Autodesk Inventor part; units mm, degrees
ref_plane "YZ Plane" through (0, 0, 0) normal (1, 0, 0) x (0, 1, 0)
ref_plane "XZ Plane" through (0, 0, 0) normal (0, 1, 0) x (-1, 0, 0)
ref_plane "XY Plane" through (0, 0, 0) normal (0, 0, 1) x (1, 0, 0)
sketch "Эскиз1" plane through (0, 0, 0) normal (0, 1, 0) x (-1, 0, 0)
  line L0 (0, 0) -> (-19.5, 0)
  line L1 (-19.5, 0) -> (-19.5, -40.5)
  line L2 (-19.5, -40.5) -> (0, -40.5)
  line L3 (0, -40.5) -> (0, 0)
  line L4 (-19.5, -40.5) -> (-19.5, -45.5)
  line L5 (-19.5, -45.5) -> (-15, -45.5)
  line L6 (0, -45.5) -> (-4.5, -45.5)
  line L7 (-4.5, -45.5) -> (-15, -45.5)
  line L8 (0, -40.5) -> (-19.5, -40.5)
  line L9 (-19.5, -40.5) -> (-19.5, -50.5)
  line L10 (-19.5, -50.5) -> (0, -50.5)
  line L11 (0, -50.5) -> (0, -40.5)
  line L12 (0, 0) -> (-19.5, 0)
  line L13 (-19.5, 0) -> (-19.5, 10)
  line L14 (-19.5, 10) -> (0, 10)
  line L15 (0, 10) -> (0, 0)
  line L16 (0, 5) -> (-4.5, 5)
  line L17 (-4.5, 5) -> (-15, 5)
  line L18 (-15, 5) -> (-19.5, 5)
  line L19 (-19.5, -50.5) -> (-23.5, -50.5)
  line L20 (-23.5, -50.5) -> (-23.5, 10)
  line L21 (-23.5, 10) -> (-19.5, 10)
  line L22 (-19.5, 10) -> (-19.5, -50.5)
  line L23 (0, 10) -> (4, 10)
  line L24 (4, 10) -> (4, -50.5)
  line L25 (4, -50.5) -> (0, -50.5)
  line L26 (0, -50.5) -> (0, 10)
  circle A0 centre (-4.5, -45.5) radius 1.25
  circle A1 centre (-15, -45.5) radius 1.25
  circle A2 centre (-4.5, 5) radius 1.25
  circle A3 centre (-15, 5) radius 1.25
  circle A4 centre (0, -40.5) radius 0.5
  circle A5 centre (-19.5, -40.5) radius 0.5
  circle A6 centre (0, 0) radius 0.5
  circle A7 centre (-19.5, 0) radius 0.5
  point P0 (-19, 0)
  point P1 (-0.5, 0)
  point P2 (0, -0.5)
  point P3 (0, -40)
  point P4 (-0.5, -40.5)
  point P5 (-19, -40.5)
  point P6 (-19.5, -40)
  point P7 (-19.5, -0.5)
  dimension "d0" = 19.5
  dimension "d1" = 40.5
  dimension "d2" = 5
  dimension "d3" = 4.5
  dimension "d4" = 4.5
  dimension "d5" = 10
  dimension "d6" = 10
  dimension "d7" = 4
  dimension "d8" = 4
  dimension "d9" = 2.5
  dimension "d10" = 2.5
  dimension "d11" = 2.5
  dimension "d12" = 2.5
  dimension "d16" = 1
  dimension "d17" = 1
  dimension "d18" = 1
  dimension "d19" = 1
extrude "Выдавливание1" add sketch "Эскиз1" along normal blind 7 contours A7 L13 L18 A3 L17 A2 L16 L15 A6 L0 | A7 L1 A5 L4 L9 L19 L20 L21 L13 | L15 L23 L24 L25 L11 A4 L3 A6 | L13 L14 L15 L16 A2 L17 A3 L18 | L2 A4 L11 L6 A0 L7 A1 L5 L4 A5 | L5 A1 L7 A0 L6 L11 L10 L9
fillet "Сопряжение1" radius 0.4 8 edges at (0, 3.5, -0.5) (0.5, 3.5, 0) (0, 3.5, -40) (0.5, 3.5, -40.5) (19.5, 3.5, -40) (19, 3.5, -40.5) (19.5, 3.5, -0.5) (19, 3.5, 0)
sketch "Эскиз2" plane through (0, 7, 0) normal (0, 1, 0) x (1, 0, 0)
  circle A0 centre (4.5, -5) radius 1.25
  line L0 (4.5, -5) -> (4.5, -2.3)
  circle A1 centre (15, 45.5) radius 1.25
  line L1 (15, 45.5) -> (15, 42.8)
  line L2 (13.4412, 42.8) -> (11.8823, 45.5)
  line L3 (11.8823, 45.5) -> (13.4412, 48.2)
  line L4 (13.4412, 48.2) -> (16.5588, 48.2)
  line L5 (16.5588, 48.2) -> (18.1177, 45.5)
  line L6 (18.1177, 45.5) -> (16.5588, 42.8)
  line L7 (16.5588, 42.8) -> (13.4412, 42.8)
  circle A2 centre (4.5, 45.5) radius 1.25
  line L8 (2.9412, 42.8) -> (1.3823, 45.5)
  line L9 (1.3823, 45.5) -> (2.9412, 48.2)
  line L10 (2.9412, 48.2) -> (6.0588, 48.2)
  line L11 (6.0588, 48.2) -> (7.6177, 45.5)
  line L12 (7.6177, 45.5) -> (6.0588, 42.8)
  line L13 (6.0588, 42.8) -> (2.9412, 42.8)
  line L14 (6.0588, -2.3) -> (7.6177, -5)
  line L15 (7.6177, -5) -> (6.0588, -7.7)
  line L16 (6.0588, -7.7) -> (2.9412, -7.7)
  line L17 (2.9412, -7.7) -> (1.3823, -5)
  line L18 (1.3823, -5) -> (2.9412, -2.3)
  line L19 (2.9412, -2.3) -> (6.0588, -2.3)
  circle A3 centre (15, -5) radius 1.25
  line L20 (16.5588, -2.3) -> (18.1177, -5)
  line L21 (18.1177, -5) -> (16.5588, -7.7)
  line L22 (16.5588, -7.7) -> (13.4412, -7.7)
  line L23 (13.4412, -7.7) -> (11.8823, -5)
  line L24 (11.8823, -5) -> (13.4412, -2.3)
  line L25 (13.4412, -2.3) -> (16.5588, -2.3)
  point P0 (0, 0)
  point P1 (4.5, 42.8)
  point P2 (15, -2.3)
  dimension "d21" = 2.7
  dimension "d22" = 2.7
extrude "Выдавливание2" cut sketch "Эскиз2" against normal blind 3.5 contours A0 | L19 L14 L15 L16 L17 L18 | A1 | L7 L2 L3 L4 L5 L6 | A2 | L8 L9 L10 L11 L12 L13 | A3 | L20 L21 L22 L23 L24 L25
properties part number "vydacha"
Read the model definition and answer for the solid it produces. Units are mm, in the model's axes. A direction names the side the tool comes from. Coordinates: 2 decimals unless noted, no trailing zeros. Loops run counter-clockwise (first coordinate to the right, second up) from the corner with the lowest first, then second, coordinate; pieces in that order, holes last. Notation, with made-up numbers: (37, 89.25) -> (81, 89.25) arc R10 cw to (81, 95.25) -> close; hole circle Ø11 at (-4.5, 46.25). An arc over 180 degrees is marked (long way). Return JSON: item names as keys, results as strings.
Item 1: Find section A-A (z = -5.5). Determine the outline of the cut face in (x, y).
Answers:
{"outline": "(-4, 0) -> (0, 0) -> (0, 7) -> (-4, 7) -> close; (19.5, 0) -> (23.5, 0) -> (23.5, 7) -> (19.5, 7) -> close"}
Item 2: Flat-ended cylindrical pins translate along their axes: P1, Ø1.5, axis at x = 4.5, z = 5, coming from the +Y side; P2, Ø6, axis at x = 3, z = 6, coming from the +Y side; P3, Ø3, axis at x = 4.5, z = -45.5, coming from the +Y side. Find the tip coordinate at first contact, or state that the pin passes through.
Answers:
{"P1": "passes through", "P2": "stops at y = 7", "P3": "stops at y = 3.5"}
Item 3: For a pull along X with two mould halves and no side action, classify faces 1 (the flat face through (-2, 0, -13)), 2 (the flat face through (15, 5, 2.3)), 3 (the flat face through (23.5, 3, -21)) as +X half, -X half, draft (parallel to the pull), parting line (faces both ways), or undercut.
Answers:
{"face 1": "draft", "face 2": "undercut", "face 3": "+X half"}
Item 4: Find section C-C (y = 4.25). Count the separate pieces of the cut face and the enclosed holes in it, plus the area to 3 significant figures.
Answers:
{"separate pieces": "1", "enclosed holes": "5", "area": "771 mm2"}
Item 5: Find the intervals of material crossed by probe 1 along X at (y, z) = (1.85, 5); probe 2 along Z at (x, y) = (15, 0.9); probe 3 along Z at (x, y) = (11.75, 6), in increasing order.
Answers:
{"probe 1": "x = -4 to 3.25, 5.75 to 13.75, 16.25 to 23.5", "probe 2": "z = -50.5 to -46.75, -44.25 to -40.5, 0 to 3.75, 6.25 to 10", "probe 3": "z = -50.5 to -40.5, 0 to 10"}
Item 6: For faces 4 (the flat face through (16, 3.5, -44)), 5 (the flat face through (0, 3, -21)), determine the directions among +Z, -Z, +X, -X, +Y, -Y from which every point of the face is accessible in a straight line to the end or side of a thin tool.
Answers:
{"face 4": "+Y", "face 5": "+Y, -Y"}
Item 7: Find section B-B (x = 4.5). Determine the outline of the cut face in (y, z).
Answers:
{"outline": "(0, -50.5) -> (7, -50.5) -> (7, -48.2) -> (3.5, -48.2) -> (3.5, -46.75) -> (0, -46.75) -> close; (0, -44.25) -> (3.5, -44.25) -> (3.5, -42.8) -> (7, -42.8) -> (7, -40.5) -> (0, -40.5) -> close; (0, 0) -> (7, 0) -> (7, 2.3) -> (3.5, 2.3) -> (3.5, 3.75) -> (0, 3.75) -> close; (0, 6.25) -> (3.5, 6.25) -> (3.5, 7.7) -> (7, 7.7) -> (7, 10) -> (0, 10) -> close"}
